from build123d import *

# Parameters (mm, degrees)
SKETCH1_R           = 15
BOSS_EXTRUDE1_DEPTH = 25
SKETCH2_R           = 4
CUT_EXTRUDE1_DEPTH  = 25


with BuildPart() as part:
    # Sketch1 → Boss-Extrude1 (new body)
    with BuildSketch(Plane.XY):
        Circle(SKETCH1_R)
    extrude(amount=BOSS_EXTRUDE1_DEPTH)

    # Sketch2 → Cut-Extrude1 (cut)
    with BuildSketch(Plane.XY.offset(25)):
        with BuildLine():
            ThreePointArc((10.42269345, 9.106766731), (6.005266621, 12.47006463), (0.621513859, 13.826766056))
            Line((0.621513859, 13.826766056), (0.621513859, 4.961221676))
            ThreePointArc((0.621513859, 4.961221676), (2.169418696, 4.50484434), (3.491331745, 3.579190222))
            Line((3.491331745, 3.579190222), (10.42269345, 9.106766731))
        make_face()
        with BuildLine():
            Line((-0.621513859, 4.961221676), (-0.621513859, 13.826766056))
            ThreePointArc((-0.621513859, 13.826766056), (-6.005266621, 12.47006463), (-10.42269345, 9.106766731))
            Line((-10.42269345, 9.106766731), (-3.491331745, 3.579190222))
            ThreePointArc((-3.491331745, 3.579190222), (-2.169418696, 4.50484434), (-0.621513859, 4.961221676))
        make_face()
        Circle(SKETCH2_R)
        with BuildLine():
            ThreePointArc((13.618400008, -2.470813687), (13.493711611, 3.079851621), (11.197708557, 8.134928527))
            Line((11.197708557, 8.134928527), (4.266346851, 2.607352018))
            ThreePointArc((4.266346851, 2.607352018), (4.874639561, 1.11260467), (4.975133335, -0.498044472))
            Line((4.975133335, -0.498044472), (13.618400008, -2.470813687))
        make_face()
        with BuildLine():
            Line((-4.266346851, 2.607352018), (-11.197708557, 8.134928527))
            ThreePointArc((-11.197708557, 8.134928527), (-13.493711611, 3.079851621), (-13.618400008, -2.470813687))
            Line((-13.618400008, -2.470813687), (-4.975133335, -0.498044472))
            ThreePointArc((-4.975133335, -0.498044472), (-4.874639561, 1.11260467), (-4.266346851, 2.607352018))
        make_face()
        with BuildLine():
            ThreePointArc((6.559173595, -12.187821003), (10.821116537, -8.629552476), (13.341800319, -3.682676106))
            Line((13.341800319, -3.682676106), (4.698533646, -1.70990689))
            ThreePointArc((4.698533646, -1.70990689), (3.909157412, -3.117449009), (2.71255805, -4.20024152))
            Line((2.71255805, -4.20024152), (6.559173595, -12.187821003))
        make_face()
        with BuildLine():
            Line((-4.698533646, -1.70990689), (-13.341800319, -3.682676106))
            ThreePointArc((-13.341800319, -3.682676106), (-10.821116537, -8.629552476), (-6.559173595, -12.187821003))
            Line((-6.559173595, -12.187821003), (-2.71255805, -4.20024152))
            ThreePointArc((-2.71255805, -4.20024152), (-3.909157412, -3.117449009), (-4.698533646, -1.70990689))
        make_face()
        with BuildLine():
            ThreePointArc((-5.439244318, -12.727150518), (0, -13.840727548), (5.439244318, -12.727150518))
            Line((5.439244318, -12.727150518), (1.592628773, -4.739571034))
            ThreePointArc((1.592628773, -4.739571034), (0, -5), (-1.592628773, -4.739571034))
            Line((-1.592628773, -4.739571034), (-5.439244318, -12.727150518))
        make_face()
    extrude(amount=-CUT_EXTRUDE1_DEPTH, mode=Mode.SUBTRACT)


solid = part.part
Work out the finished part from the listing and answer in its coordinate system (mm). A direction names the side the tool comes from. Round coordinates to 2 decimals unless told otherwise and drop trailing zeros. Write each loop counter-clockwise with the first axis right and the second up, starting at its lowest first coordinate (ties: lowest second). Pieces come first, ordered by that corner, then holes. Notation, with made-up numbers: (85, 28) - (110, 28) arc R13 cw to (110, 35) - close; hole circle Ø11 at (-34, 29). An arc over 180 degrees is marked (long way). Answer in a Markdown table with one row per item. Add a question column.
1. The mould has two halves that part along X. Classify faces 1 (the flat face through (-0.1, -4.4, 25)), 2 (the cylindrical face through (4, -3, 13)), 3 (the cylindrical face through (-14.985, 0.66, 12.325)): +X half, -X half, draft (parallel to the pull), parting line (faces both ways), or undercut.
2. For faces 4 (the cylindrical face through (0, -5, 13)), 5 (the flat face through (-0.1, -4.4, 0)), determine the directions among +Z, -Z, +X, -X, +Y, -Y from which every point of the face is accessible in a straight line to the end or side of a thin tool.
3. Find the intervals of material crossed by line 1 along Y through (x, z) = (0, 8.25); line 2 along Y through (x, z) = (-6.25, 8.75); line 3 along X through (y, z) = (5, 21.5), in increasing order. Write a range as from..to.
4. A cutting plane is placed at C-C, the plane z = 12.5. Count the separate pieces of the cut face and the enclosed holes in it, and give its area (3 significant figures).
5. A cutting plane is placed at D-D, the plane y = 11.25. Determine the outline of the cut face in (x, z).
6. Given pin 1 (1.5 mm diameter, centred on y = -6.5, z = 12, fed in from -X); pin 2 (1.5 mm diameter, centred on x = -4.5, z = 22, fed in from +Y); pin 3 (5 mm diameter, centred on x = -11, z = 10, fed in from -Y), each flat-ended and moving along its own axis, determine where each tip first touches the part or whether it passes through.
7. A cutting plane is placed at B-B, the plane y = 0. Determine the outline of the cut face in (x, z).
8. A cutting plane is placed at A-A, the plane x = 0. Determine the outline of the cut face in (y, z), and give its area (3 significant figures).
Worked out:
| question | item | result |
|---|---|---|
| 1 | face 1 | draft |
| 1 | face 2 | undercut |
| 1 | face 3 | parting line |
| 2 | face 4 | +Z, -Z |
| 2 | face 5 | -Z, +X, -X, +Y, -Y |
| 3 | line 1 | -15..-13.84, -5..-4, 4..15 |
| 3 | line 2 | -13.64..-11.55, -2.06..-0.79, 4.19..5.78, 12.35..13.64 |
| 3 | line 3 | -14.14..-12.91, -7.27..-5.27, -0.62..0.62, 5.27..7.27, 12.91..14.14 |
| 4 | separate pieces | 1 |
| 4 | enclosed holes | 8 |
| 4 | area | 210 mm^2 |
| 5 | outline | (-9.92, 0) - (-8.06, 0) - (-8.06, 25) - (-9.92, 25) - close; (-0.62, 0) - (0.62, 0) - (0.62, 25) - (-0.62, 25) - close; (8.06, 0) - (9.92, 0) - (9.92, 25) - (8.06, 25) - close |
| 6 | pin 1 | x = -13.85 |
| 6 | pin 2 | y = 14.52 |
| 6 | pin 3 | y = -12.36 |
| 7 | outline | (-15, 0) - (-13.84, 0) - (-13.84, 25) - (-15, 25) - close; (-5, 0) - (-4, 0) - (-4, 25) - (-5, 25) - close; (4, 0) - (5, 0) - (5, 25) - (4, 25) - close; (13.84, 0) - (15, 0) - (15, 25) - (13.84, 25) - close |
| 8 | outline | (-15, 0) - (-13.84, 0) - (-13.84, 25) - (-15, 25) - close; (-5, 0) - (-4, 0) - (-4, 25) - (-5, 25) - close; (4, 0) - (15, 0) - (15, 25) - (4, 25) - close |
| 8 | area | 329 mm^2 |
